from build123d import *

# Parameters (mm, degrees)
F0_R     = 1.5
F1_DEPTH = 2


with BuildPart() as f1:
    # F0 (on Front) → F1 (new body)
    with BuildSketch(Plane.XZ):
        with BuildLine():
            Line((34.5, 17), (3.5, 17))
            ThreePointArc((3.5, 17), (2.085786, 16.414214), (1.5, 15))
            Line((1.5, 15), (1.5, 0))
            Line((1.5, 0), (36.5, 0))
            Line((36.5, 0), (36.5, 15))
            ThreePointArc((36.5, 15), (35.914214, 16.414214), (34.5, 17))
        make_face()
        with BuildLine():
            ThreePointArc((7, 5), (4, 8), (7, 11))
            Line((7, 11), (31, 11))
            ThreePointArc((31, 11), (34, 8), (31, 5))
            Line((31, 5), (7, 5))
        make_face(mode=Mode.SUBTRACT)
        with Locations((9, 14)):
            Circle(F0_R, mode=Mode.SUBTRACT)
        with Locations((29, 14)):
            Circle(F0_R, mode=Mode.SUBTRACT)
    extrude(amount=F1_DEPTH)


solid = f1.part
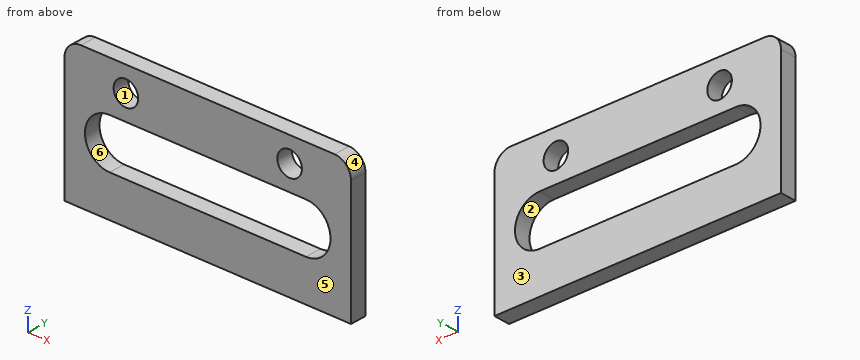
Verification items for the finished model (mm, model axes). Face numbers are marked on the shaded views. A direction names the side the tool comes from. Round coordinates to 2 decimals unless told otherwise and drop trailing zeros. Order: outer loops, then holes, each group sorted by start corner. A loop starts at its lowest first (then second) coordinate and runs counter-clockwise, first axis right, second up. Notation, with made-up numbers: (-31.5, 5.5) -> (-8.5, 5.5) arc R20 cw to (-8.5, 26.5) -> close; hole circle Ø8 at (-30, 81). An arc over 180 degrees is marked (long way). Put each result on its own line as item: value.
1) Section check D-D (z = 8). Record the cut outline in (x, y).
Final values:
outline: (1.5, -2) -> (4, -2) -> (4, 0) -> (1.5, 0) -> close; (34, -2) -> (36.5, -2) -> (36.5, 0) -> (34, 0) -> close
2) Mould release check, pull along Z, two halves, no side actions. Record for the marked faces 1, 2, 3 and 4: +Z half, -Z half, draft (parallel to the pull), parting line (faces both ways), or undercut.
Final values:
face 1: undercut
face 2: undercut
face 3: draft
face 4: +Z half
3) Section check B-B (x = 29). Record the cut outline in (y, z).
Final values:
outline: (-2, 0) -> (0, 0) -> (0, 5) -> (-2, 5) -> close; (-2, 11) -> (0, 11) -> (0, 12.5) -> (-2, 12.5) -> close; (-2, 15.5) -> (0, 15.5) -> (0, 17) -> (-2, 17) -> close
4) Section check A-A (z = 14). Record the cut outline in (x, y), then the cut area to 3 significant figures.
Final values:
outline: (1.5, -2) -> (7.5, -2) -> (7.5, 0) -> (1.5, 0) -> close; (10.5, -2) -> (27.5, -2) -> (27.5, 0) -> (10.5, 0) -> close; (30.5, -2) -> (36.5, -2) -> (36.5, 0) -> (30.5, 0) -> close
area: 58.0 mm^2
5) Set-up check for the marked faces 5 and 6: record each of +Z, -Z, +X, -X, +Y, -Y from which the full face is reachable in a straight line by a thin tool's end or side.
Final values:
face 5: +Z, -Z, +X, -X, -Y
face 6: +Y, -Y
6) Depth check by flat-ended pin: pin 1 (2.5 mm diameter, centred on x = 9, z = 14, fed in from -Y). Enter the tip coordinate at first touch or a pass-through.
Final values:
pin 1: passes through
7) Material ranges on line 1 (Z direction, x = 9, y = -0.75); line 2 (Z direction, x = 25.5, y = -0.6); line 3 (X direction, y = -0.4, z = 15), recorded low to high.
Final values:
line 1: z = 0 to 5, 11 to 12.5, 15.5 to 17
line 2: z = 0 to 5, 11 to 17
line 3: x = 1.5 to 7.88, 10.12 to 27.88, 30.12 to 36.5
8) Section check C-C (x = 17). Record the cut outline in (y, z).
Final values:
outline: (-2, 0) -> (0, 0) -> (0, 5) -> (-2, 5) -> close; (-2, 11) -> (0, 11) -> (0, 17) -> (-2, 17) -> close
